Part model, mm, in its own coordinate system. Face numbers are marked on the shaded views. A direction names the side the tool comes from. Give positions to 0.01 mm unless a question says otherwise; leave off trailing zeros. Order: outer loops, then holes, each group sorted by start corner. A loop starts at its lowest first (then second) coordinate and runs counter-clockwise, first axis right, second up. Notation, with made-up numbers: (2.25, 67) - (31.25, 67) arc R14 cw to (31.25, 92) - close; hole circle Ø5 at (-24.75, 6). An arc over 180 degrees is marked (long way). One line per item, written item: value.
```python
from build123d import *

# Parameters (mm, degrees)
F0_W     = 152.4
F0_H     = 127
F0_R     = 12.7
F1_DEPTH = 20.32
F2_DEPTH = 52.07
F3_DEPTH = 52.07


with BuildPart() as f1:
    # F0 (on Front) → F1 (new body)
    with BuildSketch(Plane.XZ):
        with Locations((-31.75, 0)):
            Rectangle(F0_W, F0_H)
        Polygon((-6.35, -21.997045), (6.35, 0), (19.05, -21.997045), align=None, mode=Mode.SUBTRACT)
        with Locations((-82.55, 0)):
            Circle(F0_R, mode=Mode.SUBTRACT)
        Polygon((-22.225, 9.525), (-22.225, 0), (-22.225, -9.525), (-41.275, -9.525), (-41.275, 0), (-41.275, 9.525), align=None, mode=Mode.SUBTRACT)
    extrude(amount=F1_DEPTH)

    # F0 (on Front) → F2 (join)
    with BuildSketch(Plane.XZ):
        with Locations((-82.55, 0)):
            Circle(F0_R)
    extrude(amount=F2_DEPTH)

    # F0 (on Front) → F3 (join)
    with BuildSketch(Plane.XZ):
        Polygon((-22.225, -9.525), (-22.225, 0), (-31.75, 0), (-41.275, 0), (-41.275, -9.525), align=None)
        Polygon((-31.75, 0), (-22.225, 0), (-22.225, 9.525), (-41.275, 9.525), (-41.275, 0), align=None)
    extrude(amount=F3_DEPTH)


solid = f1.part
```
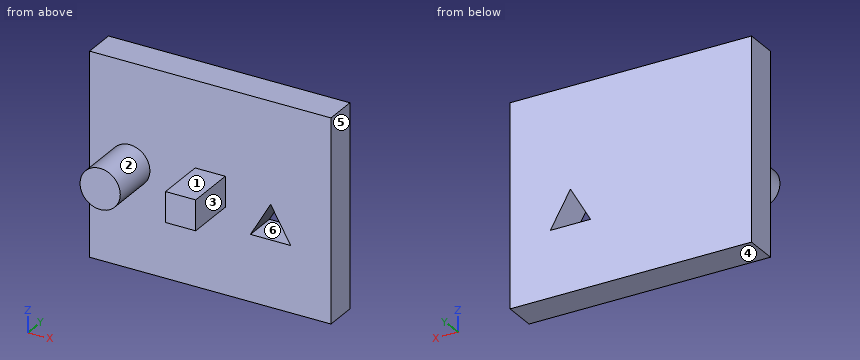
1) Mould opens along X. For the marked faces 4, 5 and 6 say: released by +X, released by -X, zero draft, split by the parting line, or undercut.
Outcome:
face 4: zero draft
face 5: released by +X
face 6: undercut
2) Cut at B-B, the plane y = -36. Give the cut face in (x, z) (3 decimals), then the cut area to 3 significant figures.
Outcome:
outline: circle Ø25.4 at (-82.55, 0); (-41.275, -9.525) - (-22.225, -9.525) - (-22.225, 9.525) - (-41.275, 9.525) - close
area: 870 mm^2
3) Cut at A-A, the plane x = -82.55. Give the cut face in (y, z).
Outcome:
outline: (-52.07, -12.7) - (-20.32, -12.7) - (-20.32, -63.5) - (0, -63.5) - (0, 63.5) - (-20.32, 63.5) - (-20.32, 12.7) - (-52.07, 12.7) - close
4) Cut at D-D, the plane x = -26.5. Give the cut face in (y, z) (3 decimals).
Outcome:
outline: (-52.07, -9.525) - (-20.32, -9.525) - (-20.32, -63.5) - (0, -63.5) - (0, 63.5) - (-20.32, 63.5) - (-20.32, 9.525) - (-52.07, 9.525) - close
5) Drill centre lines: line 1 along Y through (x, z) = (-26, -27); line 2 along Z through (x, y) = (-38, -21.5) (3 decimals); line 3 along X through (y, z) = (-42, 9) (3 decimals). Where is each one in solid material? Low to high. Write a range as from..to.
Outcome:
line 1: y = -20.32..0
line 2: z = -9.525..9.525
line 3: x = -91.51..-73.59, -41.275..-22.225
6) Which spindle directions (+Z, -Z, +X, -X, +Y, -Y) get a long thin tool onto all of the face, cutting with end or side? Do the marked faces 1, 2 and 3. Say none if no direction does.
Outcome:
face 1: +Z, +X, -Y
face 2: -Y
face 3: +Z, -Z, +X, -Y
7) Cut at C-C, the plane z = 2. Give the cut face in (x, y) (3 decimals), then the cut area to 3 significant figures.
Outcome:
outline: (-107.95, -20.32) - (-95.092, -20.32) - (-95.092, -52.07) - (-70.008, -52.07) - (-70.008, -20.32) - (-41.275, -20.32) - (-41.275, -52.07) - (-22.225, -52.07) - (-22.225, -20.32) - (44.45, -20.32) - (44.45, 0) - (-107.95, 0) - close
area: 4,500 mm^2
8) Pin check, flat tips, straight feed: pin 1 (6 mm diameter, centred on y = -46, z = -12.5, fed in from -X); pin 2 (15 mm diameter, centred on y = -43.5, z = 4, fed in from +X) (3 decimals); pin 3 (4 mm diameter, centred on x = -87.5, z = 21, fed in from -Y). Stop position of each tip, or through.
Outcome:
pin 1: stops at x = -90.98
pin 2: stops at x = -22.225
pin 3: stops at y = -20.32
